Check sheet for the modelled part. Datum: model origin and axes. Units: mm. Face numbers are marked on the shaded views. A direction names the side the tool comes from. Round coordinates to 2 decimals unless told otherwise and drop trailing zeros. Loops run counter-clockwise (first coordinate to the right, second up) from the corner with the lowest first, then second, coordinate; pieces in that order, holes last. Notation, with made-up numbers: (35, 73.25) - (56, 73.25) arc R15 ccw to (56, 90.25) - close; hole circle Ø7 at (61, 14). An arc over 180 degrees is marked (long way). Put each result on its own line as item: value.
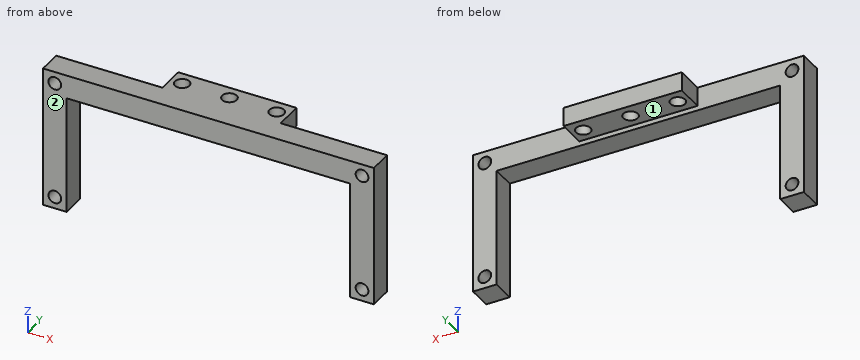
```python
from build123d import *

# Parameters (mm, degrees)
SKETCH1_W           = 70
SKETCH1_H           = 30
BOSS_EXTRUDE1_DEPTH = 5
SKETCH2_R           = 1.35
CUT_EXTRUDE1_DEPTH  = 6
SKETCH3_W           = 25
SKETCH3_H           = 4
BOSS_EXTRUDE2_DEPTH = 6
SKETCH4_R           = 1.55
CUT_EXTRUDE2_DEPTH  = 5
SKETCH5_W           = 60
SKETCH5_H           = 25
CUT_EXTRUDE3_DEPTH  = 6


with BuildPart() as part:
    # Sketch1 → Boss-Extrude1 (new body)
    with BuildSketch(Plane(origin=(0, 0, 0), x_dir=(1, 0, 0), z_dir=(0, 1, 0))):
        Rectangle(SKETCH1_W, SKETCH1_H)
    extrude(amount=BOSS_EXTRUDE1_DEPTH)

    # Sketch2 → Cut-Extrude1 (cut, through all)
    with BuildSketch(Plane(origin=(0, 5, 0), x_dir=(1, 0, 0), z_dir=(0, 1, 0))):
        with Locations((-32.5, 12.5)):
            Circle(SKETCH2_R)
        with Locations((32.5, 12.5)):
            Circle(SKETCH2_R)
        with Locations((-32.5, -12.5)):
            Circle(SKETCH2_R)
        with Locations((32.5, -12.5)):
            Circle(SKETCH2_R)
    extrude(amount=-CUT_EXTRUDE1_DEPTH, mode=Mode.SUBTRACT)

    # Sketch3 → Boss-Extrude2 (add)
    with BuildSketch(Plane(origin=(0, 5, 0), x_dir=(1, 0, 0), z_dir=(0, 1, 0))):
        with Locations((0, -13)):
            Rectangle(SKETCH3_W, SKETCH3_H)
    extrude(amount=BOSS_EXTRUDE2_DEPTH)

    # Sketch4 → Cut-Extrude2 (cut, through all)
    with BuildSketch(Plane(origin=(0, 0, 11), x_dir=(-1, 0, 0), z_dir=(0, 0, -1))):
        with Locations((-10, 8)):
            Circle(SKETCH4_R)
        with Locations((0, 8)):
            Circle(SKETCH4_R)
        with Locations((10, 8)):
            Circle(SKETCH4_R)
    extrude(amount=-CUT_EXTRUDE2_DEPTH, mode=Mode.SUBTRACT)

    # Sketch5 → Cut-Extrude3 (cut, through all)
    with BuildSketch(Plane(origin=(0, 5, 0), x_dir=(1, 0, 0), z_dir=(0, 1, 0))):
        with Locations((0, 2.5)):
            Rectangle(SKETCH5_W, SKETCH5_H)
    extrude(amount=-CUT_EXTRUDE3_DEPTH, mode=Mode.SUBTRACT)


solid = part.part
```
Item 1: Section check D-D on x = 10.5. Enter the section's corners in (y, z), then the cut area to 3 significant figures.
Filled sheet:
outline: (0, 10) - (5, 10) - (5, 11) - (6.53, 11) - (6.53, 15) - (0, 15) - close; (9.47, 11) - (11, 11) - (11, 15) - (9.47, 15) - close
area: 37.3 mm²
Item 2: Section check B-B on x = 32.5. Enter the section's corners in (y, z), then the cut area to 3 significant figures.
Filled sheet:
outline: (0, -15) - (5, -15) - (5, -13.85) - (0, -13.85) - close; (0, -11.15) - (5, -11.15) - (5, 11.15) - (0, 11.15) - close; (0, 13.85) - (5, 13.85) - (5, 15) - (0, 15) - close
area: 123 mm²
Item 3: Section check C-C on z = -4.25. Enter the section's corners in (x, y).
Filled sheet:
outline: (-35, 0) - (-30, 0) - (-30, 5) - (-35, 5) - close; (30, 0) - (35, 0) - (35, 5) - (30, 5) - close
Item 4: Tool access check on the marked faces 1 and 2. Record the directions out of +Z, -Z, +X, -X, +Y, -Y that give a thin tool (end or side, any length) a straight path to the whole face; none if there is none.
Filled sheet:
face 1: -Z, +X, -X, +Y
face 2: +Z, -Z, +X, -X, -Y
Item 5: Thickness scan on line 1 (Z direction, x = 32.5, y = 1.65); line 2 (X direction, y = 1.1, z = -12.5); line 3 (X direction, y = 4.75, z = 3.5). Record the ranges inside material, lowest first. Write a range as from..to.
Filled sheet:
line 1: -15..-13.85, -11.15..11.15, 13.85..15
line 2: -35..-33.85, -31.15..-30, 30..31.15, 33.85..35
line 3: -35..-30, 30..35
Item 6: Section check A-A on x = -10. Enter the section's corners in (y, z).
Filled sheet:
outline: (0, 10) - (5, 10) - (5, 11) - (6.45, 11) - (6.45, 15) - (0, 15) - close; (9.55, 11) - (11, 11) - (11, 15) - (9.55, 15) - close
Item 7: Go/stop test with flat-tipped pins: pin 1 (5 mm diameter, centred on x = -4.5, y = 6.5, fed in from -Z); pin 2 (4.5 mm diameter, centred on y = 7.5, z = 12.5, fed in from +X); pin 3 (2 mm diameter, centred on x = 32.5, z = -12.5, fed in from -Y); pin 4 (1.2 mm diameter, centred on y = 7.5, z = 13, fed in from -X). Record where each tip stops, or that it passes through.
Filled sheet:
pin 1: z = 10
pin 2: x = 12.5
pin 3: through
pin 4: x = -12.5
